Could you check a few things on this model? Use its own coordinates, in mm. Face numbers are marked on the shaded views. A direction names the side the tool comes from. Give positions to 0.01 mm unless a question says otherwise; leave off trailing zeros. Loops run counter-clockwise (first coordinate to the right, second up) from the corner with the lowest first, then second, coordinate; pieces in that order, holes last. Notation, with made-up numbers: (72, -30) -> (76, -30) arc R7 cw to (76, -24) -> close; hole circle Ø4 at (89.25, 13). An arc over 180 degrees is marked (long way). Write each question's results on one line, items separated by ' | '. Start each with the question number.
Q1. If we section it at A-A, the plane y = 0: List the corners of the cut face in (x, z) for me.
Q2. If I drill on line 1 along Y through (x, z) = (56.5, 18.5); line 2 along Y through (x, z) = (54, 4.5); line 3 along X through (y, z) = (-49, 29), over which ranges is the centre line in solid material (lowest first)?
Q3. If we section it at D-D, the plane x = 10: List the corners of the cut face in (y, z) for me.
Q4. If we section it at B-B, the plane x = 60: List the corners of the cut face in (y, z) for me, plus the area to 3 significant figures.
Q5. Which directions (+Z, -Z, +X, -X, +Y, -Y) give clear straight access to the entire face, cutting with the end or side of a thin tool? Please do the marked faces 4, 5 and 6.
Q6. If we section it at C-C, the plane z = 35: List the corners of the cut face in (x, y) for me, plus the area to 3 significant figures.
Q7. Will these pins go through, and if not, where does the flat tip stop? P1, Ø1.5, axis at x = -47, z = 36, coming from the -Y side; P2, Ø11.5, axis at x = 56.83, y = 0, coming from the +Z side; P3, Ø4, axis at x = -11.5, y = 37, coming from the +Z side.
Q8. We'd pull the mould along Y, two halves only. Please class the marked faces 1, 2 and 3: released by +Y, released by -Y, zero draft, split by the parting line, or undercut.
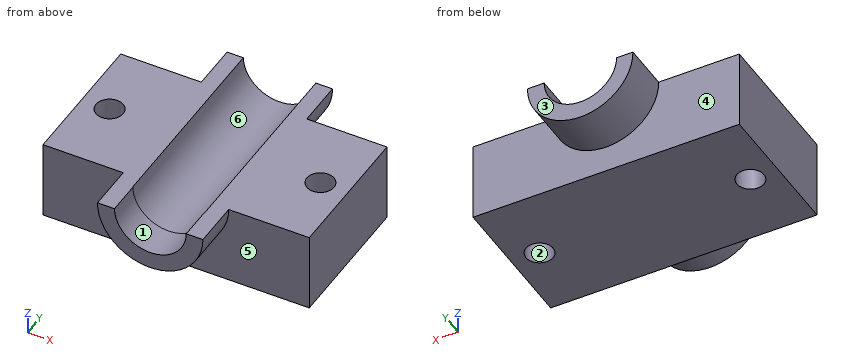
from build123d import *

# Parameters (mm, degrees)
F0_W     = 143.5509369683
F0_H     = 76.5728146038
F0_R     = 7.3255293143
F1_DEPTH = 43.18
F3_DEPTH = 25.4
F5_DEPTH = 25.4
F6_DEPTH = 83.82


with BuildPart() as f1:
    # F0 (on Top) → F1 (new body)
    with BuildSketch(Plane.XY):
        Rectangle(F0_W, F0_H)
        with Locations((-56.8299391699, 0)):
            Circle(F0_R, mode=Mode.SUBTRACT)
        with Locations((56.8299391699, 0)):
            Circle(F0_R, mode=Mode.SUBTRACT)
    extrude(amount=F1_DEPTH)

    # F2 (on face) → F3 (join)
    with BuildSketch(Plane.XZ.offset(38.2864073019)):
        with BuildLine():
            Line((-19.3430762738, 43.18), (-28.5261534154, 43.18))
            ThreePointArc((-28.5261534154, 43.18), (-0.0976910815, 14.70231059), (28.3307712525, 43.18))
            Line((28.3307712525, 43.18), (19.3430762738, 43.18))
            ThreePointArc((19.3430762738, 43.18), (0, 23.9099304509), (-19.3430762738, 43.18))
        make_face()
    extrude(amount=F3_DEPTH)

    # F4 (on face) → F5 (join)
    with BuildSketch(Plane(origin=(0, 38.2864073019, 0), x_dir=(-1, 0, 0), z_dir=(0, 1, 0))):
        with BuildLine():
            Line((-19.538462162, 43.18), (-28.5261534154, 43.18))
            ThreePointArc((-28.5261534154, 43.18), (-0.0976910815, 14.5425554008), (28.3307712525, 43.18))
            Line((28.3307712525, 43.18), (19.5384602994, 43.18))
            ThreePointArc((19.5384602994, 43.18), (-9.313e-07, 23.8160529924), (-19.538462162, 43.18))
        make_face()
    extrude(amount=F5_DEPTH)

    # F6 (cut): a face of the model
    f6_faces = [f1.faces().sort_by_distance(p)[0] for p in [
        (9.313e-07, 38.2864073019, 34.9677769674),
    ]]
    extrude(f6_faces, amount=-F6_DEPTH, mode=Mode.SUBTRACT)


solid = f1.part
Final values:
1) outline: (-71.78, 0) -> (-64.16, 0) -> (-64.16, 43.18) -> (-71.78, 43.18) -> close; (-49.5, 0) -> (49.5, 0) -> (49.5, 43.18) -> (19.54, 43.18) arc R19.54 cw to (-19.54, 43.18) -> (-49.5, 43.18) -> close; (64.16, 0) -> (71.78, 0) -> (71.78, 43.18) -> (64.16, 43.18) -> close
2) line 1: y = -38.29 to -7.32, 7.32 to 38.29 | line 2: y = -38.29 to -6.76, 6.76 to 38.29 | line 3: x = -24.77 to -13.08, 13.08 to 24.57
3) outline: (-63.69, 16.56) -> (-38.29, 16.56) -> (-38.29, 0) -> (38.29, 0) -> (38.29, 16.32) -> (63.69, 16.32) -> (63.69, 26.57) -> (-45.53, 26.57) -> (-45.53, 26.7) -> (-63.69, 26.7) -> close
4) outline: (-38.29, 0) -> (-6.6, 0) -> (-6.6, 43.18) -> (-38.29, 43.18) -> close; (6.6, 0) -> (38.29, 0) -> (38.29, 43.18) -> (6.6, 43.18) -> close | area: 2,740 mm²
5) face 4: -Z, +Y | face 5: -Z, -Y | face 6: +Z, +Y
6) outline: (-71.78, -38.29) -> (-27.34, -38.29) -> (-27.34, -63.69) -> (-17.49, -63.69) -> (-17.49, -45.53) -> (-17.66, -45.53) -> (-17.66, 63.69) -> (-27.19, 63.69) -> (-27.19, 38.29) -> (-71.78, 38.29) -> close; (17.49, -63.69) -> (27.14, -63.69) -> (27.14, -38.29) -> (71.78, -38.29) -> (71.78, 38.29) -> (27.39, 38.29) -> (27.39, 63.69) -> (17.66, 63.69) -> (17.66, -45.53) -> (17.49, -45.53) -> close; hole circle Ø14.65 at (-56.83, 0); hole circle Ø14.65 at (56.83, 0) | area: 8,930 mm²
7) P1: stops at y = -38.29 | P2: passes through | P3: stops at z = 29.23
8) face 1: zero draft | face 2: undercut | face 3: released by +Y
